Study the drawing (mm; zero at the part's minimum x, y, z) and answer. A direction names the side the tool comes from. Round coordinates to 2 decimals unless told otherwise and drop trailing zeros. Loops run counter-clockwise (first coordinate to the right, second up) from the corner with the lowest first, then second, coordinate; pieces in that order, holes last. Notation, with made-up numbers: (31.5, 76.25) - (85.5, 76.25) arc R29 cw to (85.5, 98.25) - close; hole circle Ø1 at (58, 34). An arc over 180 degrees is marked (long way). Use CSV: the item, a comma, the result in double quotes. Start each with the question number.
1. Given pin 1 Ø4 at (x, y) = (10, 3) entering from +Z; pin 2 Ø5.5 at (x, z) = (12.5, 24.5) entering from -Y; pin 3 Ø5.5 at (y, z) = (10.5, 18.5) entering from -X, each flat-ended and moving along its own axis, determine where each tip first touches the part or whether it passes through.
2. A tool of negligible diameter and unlimited length cuts with its end or side. For the marked faces 4, 5 and 6, from which of +Z, -Z, +X, -X, +Y, -Y can it reach the whole face along a straight path? Write none if from no direction.
3. Find section A-A (y = 13.5). Give the vertices of the cut face in (x, z).
4. Find section C-C (x = 20). Give the vertices of the cut face in (y, z).
5. Determine the mould class of the marked faces 1, 2 and 3 for opening direction Z: +Z half, -Z half, draft (parallel to the pull), parting line (faces both ways), or undercut.
6. Consider line 1 along Z through (x, y) = (11, 14); line 2 along X through (y, z) = (12.5, 21). Determine where each line is inside the solid, lowest interval first.
7. Find section B-B (z = 19.5). Give the vertices of the cut face in (x, y).
8. Find section D-D (y = 24). Give the vertices of the cut face in (x, z).
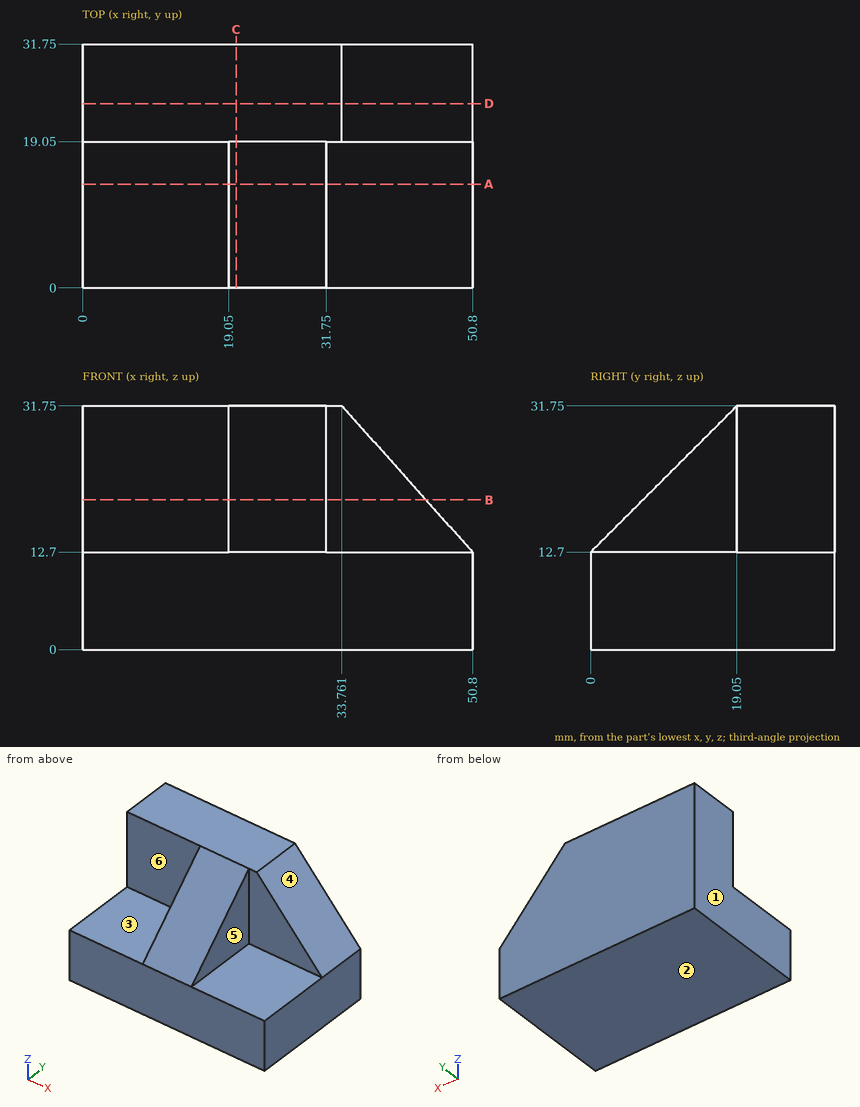
Filled sheet:
1,pin 1,"stops at z = 12.7"
1,pin 2,"stops at y = 19.05"
1,pin 3,"stops at x = 19.05"
2,face 4,"+Z, +X, +Y, -Y"
2,face 5,"+Z, +X, -Y"
2,face 6,"+Z, -X, -Y"
3,outline,"(0, 0) - (50.8, 0) - (50.8, 12.7) - (31.75, 12.7) - (31.75, 26.2) - (19.05, 26.2) - (19.05, 12.7) - (0, 12.7) - close"
4,outline,"(0, 0) - (31.75, 0) - (31.75, 31.75) - (19.05, 31.75) - (0, 12.7) - close"
5,face 1,"draft"
5,face 2,"-Z half"
5,face 3,"+Z half"
6,line 1,"z = 0 to 12.7"
6,line 2,"x = 19.05 to 31.75"
7,outline,"(0, 19.05) - (19.05, 19.05) - (19.05, 6.8) - (31.75, 6.8) - (31.75, 19.05) - (44.72, 19.05) - (44.72, 31.75) - (0, 31.75) - close"
8,outline,"(0, 0) - (50.8, 0) - (50.8, 12.7) - (33.76, 31.75) - (0, 31.75) - close"
